```python
from build123d import *

# Parameters (mm, degrees)
SKETCH_1_W          = 30
SKETCH_1_H          = 30
EXTRUDE_1_DEPTH     = 3
SKETCH_2_R          = 1.5
CUT_EXTRUDE_1_DEPTH = 3
SKETCH_3_W          = 30
SKETCH_3_H          = 3
EXTRUDE_2_DEPTH     = 27
SKETCH_5_W          = 30
SKETCH_5_H          = 30
EXTRUDE_3_DEPTH     = 3
FILLET_1_R          = 1
SKETCH_10_R         = 1.5
CUT_EXTRUDE_4_DEPTH = 3
SKETCH_11_R         = 1.5
CUT_EXTRUDE_5_DEPTH = 3


with BuildPart() as part:
    # 草图1 → 凸台-拉伸1 (new body)
    with BuildSketch(Plane.XY):
        Rectangle(SKETCH_1_W, SKETCH_1_H)
    extrude(amount=EXTRUDE_1_DEPTH)

    # 草图2 → 切除-拉伸1 (cut)
    with BuildSketch(Plane.XY.offset(3)):
        with Locations((8, 3)):
            Circle(SKETCH_2_R)
        with Locations(Location((-8, 3, 0), (0, 0, 180))):
            Circle(SKETCH_2_R)
    extrude(amount=-CUT_EXTRUDE_1_DEPTH, mode=Mode.SUBTRACT)

    # 草图3 → 凸台-拉伸2 (add)
    with BuildSketch(Plane.XY.offset(3)):
        with Locations((0, -13.5)):
            Rectangle(SKETCH_3_W, SKETCH_3_H)
    extrude(amount=EXTRUDE_2_DEPTH)

    # 草图5 → 凸台-拉伸3 (add)
    with BuildSketch(Plane.ZY.offset(15)):
        with Locations((15, 0)):
            Rectangle(SKETCH_5_W, SKETCH_5_H)
    extrude(amount=-EXTRUDE_3_DEPTH)

    # 圆角1
    fillet_1_edges = [part.edges().sort_by_distance(p)[0] for p in [
        (1.5, -12, 3),
        (-12, -12, 16.5),
    ]]
    fillet(fillet_1_edges, radius=FILLET_1_R)

    # 草图10 → 切除-拉伸4 (cut)
    with BuildSketch(Plane.XZ.offset(15)):
        with Locations((-4.393398282, 10.606601718)):
            Circle(SKETCH_10_R)
        with Locations((6.213203436, 21.213203436)):
            Circle(SKETCH_10_R)
    extrude(amount=-CUT_EXTRUDE_4_DEPTH, mode=Mode.SUBTRACT)

    # 草图11 → 切除-拉伸5 (cut)
    with BuildSketch(Plane.ZY.offset(15)):
        with Locations((23, 3)):
            Circle(SKETCH_11_R)
        with Locations(Location((7, 3, 0), (0, 0, 180))):
            Circle(SKETCH_11_R)
    extrude(amount=-CUT_EXTRUDE_5_DEPTH, mode=Mode.SUBTRACT)


solid = part.part
```
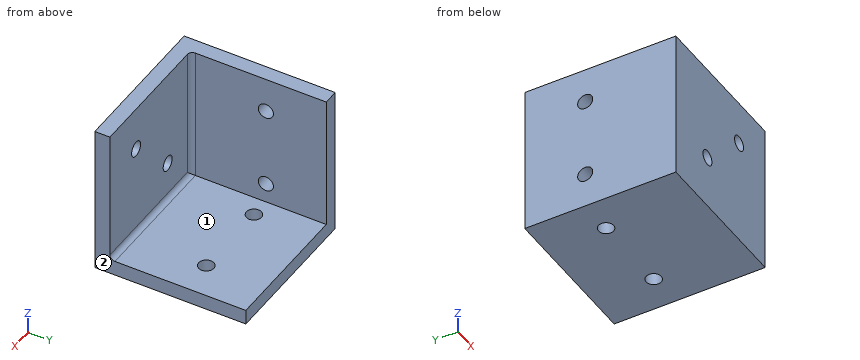
Build history of the part. All positions in model axes, mm. Face numbers are marked on the shaded views. A direction names the side the tool comes from. Round coordinates to 2 decimals unless told otherwise and drop trailing zeros. Loops run counter-clockwise (first coordinate to the right, second up) from the corner with the lowest first, then second, coordinate; pieces in that order, holes last.
Item 1: Saw through at B-B (z = 7). List the corners of the cut face in (x, y).
Item 2: Saw through at A-A (y = 3). List the corners of the cut face in (x, z), then the cut area to 3 significant figures.
Item 3: Drill centre lines: line 1 along Y through (x, z) = (-8, 0.9); line 2 along Y through (x, z) = (-7.75, 6); line 3 along Z through (x, y) = (3.25, -5.25). Where is each one in solid material? Low to high.
Item 4: Which spindle directions (+Z, -Z, +X, -X, +Y, -Y) get a long thin tool onto all of the face, cutting with end or side? Do the marked faces 1 and 2. Say none if no direction does.
Item 5: Pin check, flat tips, straight feed: P1, Ø3.5, axis at x = 8, y = 3, coming from the -Z side; P2, Ø2.5, axis at y = 3, z = 7, coming from the +X side; P3, Ø10, axis at y = 0, z = 16.5, coming from the +X side; P4, Ø6, axis at x = -8, z = 22, coming from the +Y side. Stop position of each tip, or through.
Item 6: Saw through at D-D (z = 17). List the corners of the cut face in (x, y), then the cut area to 3 significant figures.
Item 7: Saw through at C-C (x = -8). List the corners of the cut face in (y, z).
Worked answers:
1. outline: (-15, -15) - (15, -15) - (15, -12) - (-11, -12) arc R1 cw to (-12, -11) - (-12, 1.5) - (-15, 1.5) - close; (-15, 4.5) - (-12, 4.5) - (-12, 15) - (-15, 15) - close
2. outline: (-15, 0) - (-9.5, 0) - (-9.5, 3) - (-12, 3) - (-12, 5.5) - (-15, 5.5) - close; (-15, 8.5) - (-12, 8.5) - (-12, 21.5) - (-15, 21.5) - close; (-15, 24.5) - (-12, 24.5) - (-12, 30) - (-15, 30) - close; (-6.5, 0) - (6.5, 0) - (6.5, 3) - (-6.5, 3) - close; (9.5, 0) - (15, 0) - (15, 3) - (9.5, 3) - close
2. area: 135 mm2
3. line 1: y = -15 to 1.5, 4.5 to 15
3. line 2: y = -15 to -12
3. line 3: z = 0 to 3
4. face 1: +Z, +X, +Y
4. face 2: +Z, -Z, +X, +Y, -Y
5. P1: stops at z = 0
5. P2: passes through
5. P3: stops at x = -12
5. P4: stops at y = -12
6. outline: (-15, -15) - (15, -15) - (15, -12) - (-11, -12) arc R1 cw to (-12, -11) - (-12, 15) - (-15, 15) - close
6. area: 171 mm2
7. outline: (-15, 0) - (1.5, 0) - (1.5, 3) - (-11, 3) arc R1 cw to (-12, 4) - (-12, 30) - (-15, 30) - close; (4.5, 0) - (15, 0) - (15, 3) - (4.5, 3) - close
